Design review of the part built by this model. Coordinates are the model's own, in mm. Give positions to 0.01 mm unless a question says otherwise; leave off trailing zeros. Write each loop counter-clockwise with the first axis right and the second up, starting at its lowest first coordinate (ties: lowest second). Pieces come first, ordered by that corner, then holes. Notation, with made-up numbers: M 40,0 L 64,0 A31 cw 64,39 Z; hole C 15,77.25 d7. An arc over 180 degrees is marked long. Write each question's results on one line, items separated by ' | '. Start each with the question number.
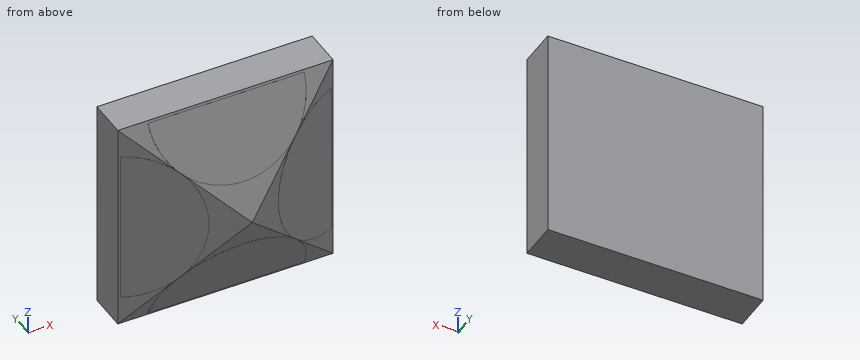
from build123d import *

# Parameters (mm, degrees)
SALIENTE_EXTRUIR1_DEPTH  = 32
CORTAR_EXTRUIR1_DEPTH    = 33
SALIENTE_EXTRUIR12_DEPTH = 0.01
SALIENTE_EXTRUIR13_DEPTH = 0.01
SALIENTE_EXTRUIR14_DEPTH = 0.01
SALIENTE_EXTRUIR15_DEPTH = 0.01


with BuildPart() as part:
    # Croquis1 → Saliente-Extruir1 (new body)
    with BuildSketch(Plane.XY):
        Polygon((-51.959662641, 8.927829358), (-51.959662641, 3.148169014), (-35.959662641, -4.290206314), (-19.959662641, 3.148169014), (-19.959662641, 8.927829358), align=None)
    extrude(amount=SALIENTE_EXTRUIR1_DEPTH)

    # Croquis2 → Cortar-Extruir1 (cut)
    with BuildSketch(Plane(origin=(-19.959662641, 0, 0), x_dir=(0, 0, -1), z_dir=(1, 0, 0))):
        Polygon((0, -4.290206314), (-16, -4.290206314), (0, 3.148169014), align=None)
        Polygon((-32, -4.290206314), (-32, 3.148169014), (-16, -4.290206314), align=None)
    extrude(amount=-CORTAR_EXTRUIR1_DEPTH, mode=Mode.SUBTRACT)

    # Croquis16 → Saliente-Extruir12 (add)
    with BuildSketch(Plane(origin=(0, -9.644179557, 4.483564205), x_dir=(-1, 0, 0), z_dir=(0, -0.906796627, 0.421568354))):
        with BuildLine():
            Line((47.568325111, -29.981567998), (36.071815605, -29.981567998))
            Line((36.071815605, -29.981567998), (24.351000171, -29.981567998))
            ThreePointArc((24.351000171, -29.981567998), (35.959662641, -18.372905528), (47.568325111, -29.981567998))
        make_face()
    extrude(amount=SALIENTE_EXTRUIR12_DEPTH)

    # Croquis17 → Saliente-Extruir13 (add)
    with BuildSketch(Plane(origin=(-8.030792992, -17.274294748, 0), x_dir=(-0.906796627, 0.421568354, 0), z_dir=(-0.421568354, -0.906796627, 0))):
        with BuildLine():
            Line((48.080668577, -16), (48.080668577, -27.608491723))
            ThreePointArc((48.080668577, -27.608491723), (36.472176853, -16), (48.080668577, -4.391508277))
            Line((48.080668577, -4.391508277), (48.080668577, -16))
        make_face()
    extrude(amount=SALIENTE_EXTRUIR13_DEPTH)

    # Croquis18 → Saliente-Extruir14 (add)
    with BuildSketch(Plane(origin=(0, 2.588676805, 1.203471855), x_dir=(-1, 0, 0), z_dir=(0, -0.906796627, -0.421568354))):
        with BuildLine():
            Line((47.567066817, 0.962202745), (35.959662641, 0.962202745))
            Line((35.959662641, 0.962202745), (24.352258465, 0.962202745))
            ThreePointArc((24.352258465, 0.962202745), (35.959662641, -10.64520143), (47.567066817, 0.962202745))
        make_face()
    extrude(amount=SALIENTE_EXTRUIR14_DEPTH)

    # Croquis19 → Saliente-Extruir15 (add)
    with BuildSketch(Plane(origin=(-4.750700642, 10.218791996, 0), x_dir=(-0.906796627, -0.421568354, 0), z_dir=(0.421568354, -0.906796627, 0))):
        with BuildLine():
            Line((17.142987404, -4.396515697), (17.142987404, -16))
            Line((17.142987404, -16), (17.142987404, -27.603484303))
            ThreePointArc((17.142987404, -27.603484303), (28.746471707, -16), (17.142987404, -4.396515697))
        make_face()
    extrude(amount=SALIENTE_EXTRUIR15_DEPTH)


solid = part.part
Q1. For pin 1 Ø3 at (x, z) = (-39.5, 23.5) entering from -Y; pin 2 Ø1.5 at (y, z) = (2, 20.5) entering from +X; pin 3 Ø3 at (x, z) = (-30, 7) entering from -Y, all flat-tipped, find the tip position at first contact; note any pin that passes through.
Q2. We need section B-B on z = 17. Write out the cut boundary in (x, y) (3 decimals), and give its area (3 significant figures).
Q3. Wall thickness on line 1 along Y through (x, z) = (-30, 24); line 2 along Y through (x, z) = (-38, 21.5); line 3 along X through (y, z) = (-0.5, 9): over which ranges is each line inside the solid? List them lowest first. Write a range as from..to.
Answer sheet:
1) pin 1: y = -1.51 | pin 2: x = -20.79 | pin 3: y = -0.81
2) outline: M -51.96,3.148 L -51.63,2.995 L -51.634,2.986 L -41.147,-1.89 L -41.143,-1.881 L -36.96,-3.825 L -34.96,-3.825 L -30.779,-1.882 L -30.775,-1.891 L -20.292,2.983 L -20.296,2.992 L -19.96,3.148 L -19.96,8.928 L -51.96,8.928 Z | area: 304 mm^2
3) line 1: -0.58..8.93 | line 2: -1.74..8.93 | line 3: -44.14..-27.78
